from build123d import *

# Parameters (mm, degrees)
SKETCH1_R                  = 24
EXTRUDE1_DEPTH             = 10
SKETCH2_R                  = 14
EXTRUDE2_DEPTH             = 46
EXTRUDE3_START             = -10
EXTRUDE3_DEPTH             = 10
F_6_0_6_DIAMETER_HOLE1_D   = 6
CIRPATTERN1_COUNT          = 8
F_25_0_25_DIAMETER_HOLE1_D = 16


# Read off the part's stored shape, not the designer's step: Extrude3
with BuildPart() as part:
    # Sketch1 → Extrude1 (new body)
    with BuildSketch(Plane.XY):
        Circle(SKETCH1_R)
    extrude(amount=EXTRUDE1_DEPTH)

    # Sketch2 → Extrude2 (add)
    with BuildSketch(Plane.XY.offset(10)):
        Circle(SKETCH2_R)
    extrude(amount=EXTRUDE2_DEPTH)

    # Extrude3 outline → Extrude3 (cut)
    with BuildSketch(Plane(origin=(0, 0, 0), x_dir=(-1, 0, 0), z_dir=(0, 0, -1)).offset(EXTRUDE3_START)):
        with BuildLine():
            Line((-20, -13.266499161), (-20, 13.266499161))
            ThreePointArc((-20, 13.266499161), (-24, 0), (-20, -13.266499161))
        make_face()
        with BuildLine():
            ThreePointArc((20, -13.266499161), (24, 0), (20, 13.266499161))
            Line((20, 13.266499161), (20, -13.266499161))
        make_face()
    extrude(amount=EXTRUDE3_DEPTH, mode=Mode.SUBTRACT)

    # Ø6.0 (6) Diameter Hole1 (through all)
    with Locations(Plane(origin=(0, 0, 0), x_dir=(-1, 0, 0), z_dir=(0, 0, -1))):
        with Locations((0, 19)):
            f_6_0_6_diameter_hole1 = Hole(F_6_0_6_DIAMETER_HOLE1_D / 2)

    # CirPattern1: Ø6.0 (6) Diameter Hole1 ×8 about axis, 2 skipped
    cirpattern1_axis = Axis((0, 0, 0), (0, 0, 1))
    add([f_6_0_6_diameter_hole1.rotate(cirpattern1_axis, i * 360 / CIRPATTERN1_COUNT) for i in range(1, CIRPATTERN1_COUNT) if i not in (2, 6)], mode=Mode.SUBTRACT)

    # Ø25.0 (25) Diameter Hole1 (through all)
    with Locations(Plane(origin=(0, 0, 0), x_dir=(-1, 0, 0), z_dir=(0, 0, -1))):
        with Locations((0, 0)):
            Hole(F_25_0_25_DIAMETER_HOLE1_D / 2)


solid = part.part
Geometry check sheet. Reference: the model listing, model coordinates, mm. A direction names the side the tool comes from. Round coordinates to 2 decimals unless told otherwise and drop trailing zeros. Order: outer loops, then holes, each group sorted by start corner. A loop starts at its lowest first (then second) coordinate and runs counter-clockwise, first axis right, second up. Notation, with made-up numbers: M 13.25,79.25 L 52.25,79.25 A22 cw 52.25,91.25 Z; hole C 13.25,52 d1. An arc over 180 degrees is marked long. Answer in a Markdown table with one row per item. Add a question column.
Item 1: Sectioned sample at C-C, the plane x = -4.5. Enter the section's corners in (y, z).
Item 2: Set-up check for faces 4 (the face through (-14, -5, 10)), 5 (the face through (-20, 0, 5)): record each of +Z, -Z, +X, -X, +Y, -Y from which the full face is reachable in a straight line by a thin tool's end or side.
Item 3: Draft check along X on faces 1 (the face through (20, 0, 5)), 2 (the face through (-15.262, -15.814, 5.07)), 3 (the face through (0, -24, 5)). Enter one of: released by +X, released by -X, zero draft, split by the parting line, or undercut.
Item 4: Depth check by flat-ended pin: pin 1 Ø5 at (y, z) = (12, 31) entering from +X; pin 2 Ø8 at (x, y) = (13.44, -13.44) entering from +Z; pin 3 Ø4 at (x, z) = (-2, 49) entering from +Y. Enter the tip coordinate at first touch or a pass-through.
Item 5: Sectioned sample at B-B, the plane y = -20. Enter the section's corners in (x, z).
Item 6: Material ranges on L1, parallel to Y at x = 2.5, z = 7; L2, parallel to Y at x = 0, z = 39; L3, parallel to X at y = -15, z = 5.5 (1 decimal), recorded low to high. Write a range as [from, to].
Item 7: Sectioned sample at A-A, the plane x = 0. Enter the section's corners in (y, z), plus the area to 3 significant figures.
Item 8: Sectioned sample at D-D, the plane z = 38. Enter the section's corners in (x, y).
Filled in:
| question | item | result |
|---|---|---|
| 1 | outline | M -23.57,0 L -6.61,0 L -6.61,56 L -13.26,56 L -13.26,10 L -23.57,10 Z; M 6.61,0 L 23.57,0 L 23.57,10 L 13.26,10 L 13.26,56 L 6.61,56 Z |
| 2 | face 4 | +Z |
| 2 | face 5 | +Z, -Z, -X, +Y, -Y |
| 3 | face 1 | released by +X |
| 3 | face 2 | undercut |
| 3 | face 3 | split by the parting line |
| 4 | pin 1 | stops at x = 10.28 |
| 4 | pin 2 | stops at z = 10 |
| 4 | pin 3 | stops at y = 14 |
| 5 | outline | M -13.27,0 L -2.83,0 L -2.83,10 L -13.27,10 Z; M 2.83,0 L 13.27,0 L 13.27,10 L 2.83,10 Z |
| 6 | L1 | y = [-23.87, -20.66], [-17.34, -7.6], [7.6, 17.34], [20.66, 23.87] |
| 6 | L2 | y = [-14, -8], [8, 14] |
| 6 | L3 | x = [-18.7, -16], [-10.9, 10.9], [16, 18.7] |
| 7 | outline | M -24,0 L -22,0 L -22,10 L -24,10 Z; M -16,0 L -8,0 L -8,56 L -14,56 L -14,10 L -16,10 Z; M 8,0 L 16,0 L 16,10 L 14,10 L 14,56 L 8,56 Z; M 22,0 L 24,0 L 24,10 L 22,10 Z |
| 7 | area | 752 mm² |
| 8 | outline | C 0,0 d28; hole C 0,0 d16 |
